Read the model definition and answer for the solid it produces. Units are mm, in the model's axes. A direction names the side the tool comes from. Coordinates: 2 decimals unless noted, no trailing zeros. Write each loop counter-clockwise with the first axis right and the second up, starting at its lowest first coordinate (ties: lowest second). Pieces come first, ordered by that corner, then holes. Notation, with made-up numbers: (-3.75, 31.5) -> (30.25, 31.5) arc R6 ccw to (30.25, 42.5) -> close; hole circle Ø5 at (58, -31). An arc over 180 degrees is marked (long way). One line per item, written item: value. Start each with the question number.
1. For faces 1 (the flat face through (8, 20.705, 6)), 2 (the flat face through (-10, -27.277, 6)), 3 (the flat face through (0, 1, 6)), 4 (the flat face through (-34.069, -1, 6)), 5 (the flat face through (32.536, 11, 6)), determine the directions among +Z, -Z, +X, -X, +Y, -Y from which every point of the face is accessible in a straight line to the end or side of a thin tool.
2. Find section A-A, the plane z = 3. Write down the section's boundary in (x, y), and give its area (3 significant figures).
3. Find section B-B, the plane y = -14. Write down the section's boundary in (x, z).
4. Find section C-C, the plane x = 10. Write down the section's boundary in (y, z), and give its area (3 significant figures).
5. For a pull along Y with two mould halves and no side action, classify faces 6 (the flat face through (22.786, 11, 6)), 7 (the flat face through (7, -24.21, 6)), 8 (the flat face through (28, 28.592, 6)) as pulls with the +Y half, pulls with the -Y half, needs draft (parallel to the pull), parting line crosses it, or undercut.
6. Find section D-D, the plane x = 24. Write down the section's boundary in (y, z).
7. Given P1, Ø1, axis at y = 12, z = 8.5, coming from the -X side; P2, Ø3, axis at x = 8, z = 4.5, coming from the -Y side; P3, Ø2.5, axis at x = -10, z = 8, coming from the +Y side, each flat-ended and moving along its own axis, determine where each tip first touches the part or whether it passes through.
8. Consider line 1 along X through (y, z) = (8, 7.75); line 2 along X through (y, z) = (-9.5, 6.75); line 3 along X through (y, z) = (23.5, 7.75). Determine where each line is inside the solid, lowest interval first.
```python
from build123d import *

# Parameters (mm, degrees)
SKETCH1_W           = 80
SKETCH1_H           = 70
BOSS_EXTRUDE1_DEPTH = 0.8
SKETCH2_W           = 9.092469125
SKETCH2_H           = 29.249268146
SKETCH2_W_2         = 16.103529653
SKETCH2_H_2         = 38.34173727
SKETCH2_W_3         = 7.887443096
SKETCH2_H_3         = 51.706571405
SKETCH2_W_4         = 9.749756049
SKETCH2_H_4         = 33.740728797
SKETCH2_W_5         = 4.546234562
SKETCH2_H_5         = 3.286434623
SKETCH2_W_6         = 11.173877719
SKETCH2_H_6         = 7.23015617
BOSS_EXTRUDE2_DEPTH = 10


with BuildPart() as part:
    # Sketch1 → Boss-Extrude1 (new, symmetric)
    with BuildSketch(Plane.XY):
        Rectangle(SKETCH1_W, SKETCH1_H)
    extrude(amount=BOSS_EXTRUDE1_DEPTH, both=True)

    # Sketch2 → Boss-Extrude2 (add)
    with BuildSketch(Plane.XY.offset(0.8)):
        with Locations((-11.995486375, 2.026634684)):
            Rectangle(SKETCH2_W, SKETCH2_H)
        with Locations((8.051764827, 1.533669491)):
            Rectangle(SKETCH2_W_2, SKETCH2_H_2)
        with Locations((-30.125650712, -0.219095641)):
            Rectangle(SKETCH2_W_3, SKETCH2_H_3)
        with Locations((27.660824745, 11.721616822)):
            Rectangle(SKETCH2_W_4, SKETCH2_H_4)
        with Locations((-9.722369093, -28.920624684)):
            Rectangle(SKETCH2_W_5, SKETCH2_H_5)
        with Locations((7.449251813, -27.825146476)):
            Rectangle(SKETCH2_W_6, SKETCH2_H_6)
    extrude(amount=BOSS_EXTRUDE2_DEPTH)


solid = part.part
```
Answer block:
1. face 1: +Z, +Y
1. face 2: +Z, -X
1. face 3: +Z, +Y, -Y
1. face 4: +Z, -X, +Y, -Y
1. face 5: +Z, +X, +Y, -Y
2. outline: (-34.07, -26.07) -> (-26.18, -26.07) -> (-26.18, 25.63) -> (-34.07, 25.63) -> close; (-16.54, -12.6) -> (-7.45, -12.6) -> (-7.45, 16.65) -> (-16.54, 16.65) -> close; (-12, -30.56) -> (-7.45, -30.56) -> (-7.45, -27.28) -> (-12, -27.28) -> close; (0, -17.64) -> (16.1, -17.64) -> (16.1, 20.7) -> (0, 20.7) -> close; (1.86, -31.44) -> (13.04, -31.44) -> (13.04, -24.21) -> (1.86, -24.21) -> close; (22.79, -5.15) -> (32.54, -5.15) -> (32.54, 28.59) -> (22.79, 28.59) -> close
2. area: 1,720 mm2
3. outline: (-40, -0.8) -> (40, -0.8) -> (40, 0.8) -> (16.1, 0.8) -> (16.1, 10.8) -> (0, 10.8) -> (0, 0.8) -> (-26.18, 0.8) -> (-26.18, 10.8) -> (-34.07, 10.8) -> (-34.07, 0.8) -> (-40, 0.8) -> close
4. outline: (-35, -0.8) -> (35, -0.8) -> (35, 0.8) -> (20.7, 0.8) -> (20.7, 10.8) -> (-17.64, 10.8) -> (-17.64, 0.8) -> (-24.21, 0.8) -> (-24.21, 10.8) -> (-31.44, 10.8) -> (-31.44, 0.8) -> (-35, 0.8) -> close
4. area: 568 mm2
5. face 6: needs draft
5. face 7: undercut
5. face 8: pulls with the +Y half
6. outline: (-35, -0.8) -> (35, -0.8) -> (35, 0.8) -> (28.59, 0.8) -> (28.59, 10.8) -> (-5.15, 10.8) -> (-5.15, 0.8) -> (-35, 0.8) -> close
7. P1: stops at x = -34.07
7. P2: stops at y = -31.44
7. P3: stops at y = 16.65
8. line 1: x = -34.07 to -26.18, -16.54 to -7.45, 0 to 16.1, 22.79 to 32.54
8. line 2: x = -34.07 to -26.18, -16.54 to -7.45, 0 to 16.1
8. line 3: x = -34.07 to -26.18, 22.79 to 32.54
